Can you work these out from the model? Positions are in its coordinate system, mm. A direction names the side the tool comes from. Give positions to 0.01 mm unless a question says otherwise; leave off trailing zeros. Order: outer loops, then holes, each group sorted by start corner. A loop starts at its lowest first (then second) coordinate and runs counter-clockwise, first axis right, second up.
Item 1: If I drill on line 1 along X through (y, z) = (-4, 7.5); line 2 along Y through (x, z) = (58.5, 0); line 3 along X through (y, z) = (11, 0), over which ranges is the centre line in solid material (lowest first)?
Item 2: I want a section at C-C, the plane x = 28.5. Write out the boundary of the cut face in (y, z), then the cut area to 3 significant figures.
Item 3: I'm going to push flat-ended pins straight in: pin 1 Ø5.5 at (x, y) = (59.55, 0) entering from +Z; pin 2 Ø4 at (x, y) = (43.5, -2) entering from +Z; pin 3 Ø2 at (x, z) = (15, -7) entering from -Y. Where does each tip first touch, or does it pass through?
Item 4: I want a section at A-A, the plane y = 0. Count the separate pieces of the cut face and the enclosed holes in it, then the cut area to 3 significant figures.
Item 5: Which directions (+Z, -Z, +X, -X, +Y, -Y) give clear straight access to the entire face, cutting with the end or side of a thin tool? Please do faces 4 (the flat face through (61.508, 9.505, -5.536)), 5 (the flat face through (57.05, 2.1, 4.3)), 6 (the cylindrical face through (3.698, -4.125, 7.687)).
Item 6: I want a section at B-B, the plane x = 59.55. Write out the boundary of the cut face in (y, z), then the cut area to 3 significant figures.
Item 7: If we mould it in two halves opening along Y, with no side actions, what happens to faces 1 (the flat face through (25, 6, 2)), 2 (the cylindrical face through (59.599, 7.91, -10.316)), 3 (the conical face through (8.12, 7.32, 0.12))? For each: +Y half, -Y half, draft (parallel to the pull), parting line (faces both ways), or undercut.
```python
from build123d import *

# Parameters (mm, degrees)
SKETCH_2_R                = 10
CUT_EXTRUDE_1_DEPTH       = 6
SKETCH_3_R                = 4.5
CUT_EXTRUDE_2_DEPTH       = 66.675737529
HOLE_START                = 11
HOLE_WIZARD_1_OUTLINE_R   = 3
HOLE_WIZARD_1_DEPTH       = 2.000000102
HOLE_START_2              = 9.836666254
HOLE_WIZARD_1_2_OUTLINE_R = 1.8
HOLE_WIZARD_1_2_DEPTH     = 1.163333746
PATTERN_CIRCULAR_1_COUNT  = 3
PATTERN_CIRCULAR_2_COUNT  = 6
CHAMFER_1_SIZE            = 1


# Read off the part's stored shape, not the designer's step: 打孔尺寸(%根据)内六角圆柱头螺钉的类型1
with BuildPart() as part:
    # 草图1 → 旋转1 (revolve)
    with BuildSketch(Plane.XY, mode=Mode.PRIVATE) as revolve_1_sk:
        Polygon((0, 0), (0, 10), (25, 10), (25, 6), (55.05, 6), (55.05, 13), (63.05, 13), (63.05, 0), align=None)
    revolve(revolve_1_sk.sketch.rotate(Axis((-26.16483903, 0, 0), (1, 0, 0)), 90), axis=Axis((-26.16483903, 0, 0), (1, 0, 0)))

    # 草图2 → 切除-拉伸1 (cut)
    with BuildSketch(Plane(origin=(63.05, 0, 0), x_dir=(0, 0, -1), z_dir=(1, 0, 0))):
        with Locations(Location((0, 0, 0), (0, 0, 180))):
            Circle(SKETCH_2_R)
    extrude(amount=-CUT_EXTRUDE_1_DEPTH, mode=Mode.SUBTRACT)

    # 草图3 → 切除-拉伸2 (cut, through all)
    with BuildSketch(Plane.ZY):
        Circle(SKETCH_3_R)
    extrude(amount=-CUT_EXTRUDE_2_DEPTH, mode=Mode.SUBTRACT)

    # 打孔尺寸(%根据)内六角圆柱头螺钉的类型1 outline → 打孔尺寸(%根据)内六角圆柱头螺钉的类型1 (cut)
    with BuildSketch(Plane.XY.offset(HOLE_START)):
        with Locations((59.55, 0)):
            Circle(HOLE_WIZARD_1_OUTLINE_R)
    hole_wizard_1 = extrude(amount=HOLE_WIZARD_1_DEPTH, mode=Mode.SUBTRACT)

    # Hole Wizard 1 2 outline → Hole Wizard 1 2 (cut)
    with BuildSketch(Plane.XY.offset(HOLE_START_2)):
        with Locations((59.55, 0)):
            Circle(HOLE_WIZARD_1_2_OUTLINE_R)
    hole_wizard_1_2 = extrude(amount=HOLE_WIZARD_1_2_DEPTH, mode=Mode.SUBTRACT)

    # 阵列(圆周)1: 打孔尺寸(%根据)内六角圆柱头螺钉的类型1, Hole Wizard 1 2 ×3 about axis
    pattern_circular_1_axis = Axis((0, 0, 0), (1, 0, 0))
    add([hole_wizard_1.rotate(pattern_circular_1_axis, i * 360 / PATTERN_CIRCULAR_1_COUNT) for i in range(1, PATTERN_CIRCULAR_1_COUNT)], mode=Mode.SUBTRACT)
    add([hole_wizard_1_2.rotate(pattern_circular_1_axis, i * 360 / PATTERN_CIRCULAR_1_COUNT) for i in range(1, PATTERN_CIRCULAR_1_COUNT)], mode=Mode.SUBTRACT)

    # 草图10 → M3 螺纹孔1 (revolve, cut)
    with BuildSketch(Plane.ZX.offset(7.5)):
        Polygon((0, 0), (0, 8.251075774), (1.25, 7.5), (1.25, 0), align=None)
    hole_wizard_m3_1 = revolve(axis=Axis((-6.35, 7.5, 0), (1, 0, 0)), mode=Mode.SUBTRACT)

    # 阵列(圆周)2: M3 螺纹孔1 ×6 about axis
    pattern_circular_2_axis = Axis((0, 0, 0), (1, 0, 0))
    for i in range(1, PATTERN_CIRCULAR_2_COUNT):
        add(hole_wizard_m3_1.rotate(pattern_circular_2_axis, i * 360 / PATTERN_CIRCULAR_2_COUNT), mode=Mode.SUBTRACT)

    # 倒角1
    chamfer_1_edges = [part.edges().sort_by_distance(p)[0] for p in [
        (55.05, 0, -13),
        (25, 0, -10),
    ]]
    chamfer(chamfer_1_edges, length=CHAMFER_1_SIZE)


solid = part.part
```
Results list:
1. line 1: x = 7.63 to 25, 55.05 to 57.05
1. line 2: y = -13 to -10, 10 to 13
1. line 3: x = 55.05 to 63.05
2. outline: circle Ø12 at (0, 0); hole circle Ø9 at (0, 0)
2. area: 49.5 mm2
3. pin 1: stops at z = 11
3. pin 2: stops at z = 6
3. pin 3: stops at y = -8
4. separate pieces: 3
4. enclosed holes: 0
4. area: 418 mm2
5. face 4: none
5. face 5: +X
5. face 6: -X
6. outline: (-12.45, -3.73) - (-11.03, -2.9) - (-10.43, -3.94) - (-9.42, -3.36) arc R10 cw to (-1.8, 9.84) - (-1.8, 11) - (-3, 11) - (-3, 12.65) arc R13 ccw to start; (-9.45, -8.92) arc R13 ccw to (9.45, -8.92) - (8.03, -8.1) - (8.63, -7.06) - (7.62, -6.48) arc R10 cw to (-7.62, -6.48) - (-8.63, -7.06) - (-8.03, -8.1) - close; (1.8, 9.84) arc R10 cw to (9.42, -3.36) - (10.43, -3.94) - (11.03, -2.9) - (12.45, -3.73) arc R13 ccw to (3, 12.65) - (3, 11) - (1.8, 11) - close
6. area: 171 mm2
7. face 1: draft
7. face 2: parting line
7. face 3: undercut
